Autodesk Fusion 360 part; units mm, degrees
sketch "main" plane through (0, 0, 0) normal (0, 1, 0) x (1, 0, 0) in component "crank-holder"
  line L0 (30, -20) -> (-30, -20)
  line L1 (-30, -20) -> (-30, 20)
  line L2 (-30, 20) -> (30, 20)
  line L3 (30, 20) -> (30, -20)
  line L4 (30, -20) -> (-30, 20) construction
  line L5 (-30, -20) -> (30, 20) construction
  circle A0 centre (0, 0) radius 4.425
  line L6 (-30, 20) -> (-50, 20) construction
  line L7 (-50, 20) -> (50, 20)
  line L8 (50, 20) -> (50, 5)
  line L9 (50, 5) -> (-50, 5)
  line L10 (-50, 5) -> (-50, 20)
  dimension "d1" = 60
  dimension "d2" = 40
  dimension "d3" = 8.85
  dimension "d4" = 20
  dimension "d5" = 100
  dimension "d6" = 15
extrude "Extrude1" add sketch "main" against normal blind 30 contours L0 L1 L3 L9 | L1 L2 L3 L7 L9 | L3 L7 L8 L9 | L1 L7 L9 L10 | A0 in component "crank-holder"
extrude "Extrude2" add sketch "main" along normal blind 8.5 contours A0 in component "crank-holder"
sketch "screws" plane through (0, 0, -5) normal (0, 0, 1) x (-1, 0, 0) in component "crank-holder"
  line L0 (30, 0) -> (50, 0)
  line L1 (50, 0) -> (50, 30)
  line L2 (50, 30) -> (30, 30)
  line L3 (30, 30) -> (30, 0)
  line L4 (50, 0) -> (30, 30) construction
  line L5 (50, 30) -> (30, 0) construction
  line L6 (-50, 0) -> (-30, 30) construction
  line L7 (-50, 30) -> (-30, 0) construction
  circle A0 centre (40, 15) radius 2.75
  circle A1 centre (-40, 15) radius 2.75
  point P0 (-50, 0)
  point P1 (-30, 30)
  point P2 (-50, 30)
  point P3 (-30, 0)
  dimension "d11" = 5.5
  dimension "d12" = 5.5
extrude "Extrude3" cut sketch "screws" against normal blind 15 contours A0 | A1 in component "crank-holder"
component "crank-holder" placed x (1, 0, 0) y (0, 1, 0) z (0, 0, 1) at (0, 0, 0)
equation "d5 = 20 mm + 60 mm + 20 mm"
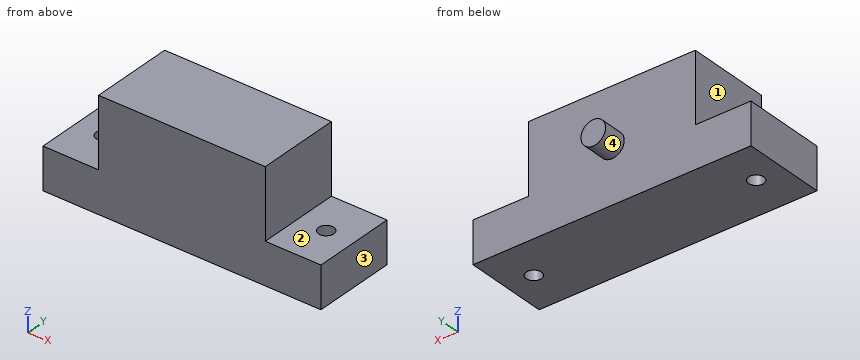
The listing builds one solid part. Answer for the finished solid, in the listing's coordinates (mm). Face numbers are marked on the shaded views. A direction names the side the tool comes from. Coordinates: 2 decimals unless noted, no trailing zeros. Loops run counter-clockwise (first coordinate to the right, second up) from the corner with the lowest first, then second, coordinate; pieces in that order, holes last. Notation, with made-up numbers: M 61,-39 L 85,-39 A14 ccw 85,-20 Z; hole C -35.75,62.5 d5. An arc over 180 degrees is marked long. Answer as a JSON object with one key per item and string values. Group by question number.
Item 1: Section C-C (z = 0) is taken. Write down the section's boundary in (x, y) (3 decimals).
Item 2: Consider L1, parallel to X at y = -15, z = -9.5; L2, parallel to Y at x = 40, z = -13.5; L3, parallel to Z at x = 37, y = -25.5. Determine where each line is inside the solid, lowest interval first.
Item 3: Which of the six approach directions +Z, -Z, +X, -X, +Y, -Y give full straight-line access (tool end or side, diameter ignored) to the marked faces 1, 2, 3 and 4?
Item 4: Section D-D (y = -7.5) is taken. Write down the section's boundary in (x, z), and give its area (3 significant figures).
Item 5: Section A-A (x = -40) is taken. Write down the section's boundary in (y, z).
Item 6: Section B-B (y = -15) is taken. Write down the section's boundary in (x, z), and give its area (4 significant figures).
Item 7: Each of these flat-tipped pins is pushed along its axis until it touches: P1, Ø6, axis at x = -35.5, y = -17.5, coming from the +Z side; P2, Ø7, axis at x = -40, y = -15, coming from the -Z side; P3, Ø10, axis at x = -3, z = -14, coming from the +Y side; P4, Ø1, axis at y = -10, z = 3.5, coming from the +X side. Where does it stop, or does it pass through?
Solved:
{
 "1": {"outline": "M -30,-30 L 30,-30 L 30,0 L 4.425,0 L 4.425,8.5 L -4.425,8.5 L -4.425,0 L -30,0 Z"},
 "2": {"L1": "x = -50 to -42.75, -37.25 to 37.25, 42.75 to 50", "L2": "y = -30 to -17.75, -12.25 to 0", "L3": "z = -20 to -5"},
 "3": {"face 1": "+Z, -X, +Y, -Y", "face 2": "+Z, +X, +Y, -Y", "face 3": "+Z, -Z, +X, +Y, -Y", "face 4": "+Y"},
 "4": {"outline": "M -50,-20 L 50,-20 L 50,-5 L 30,-5 L 30,20 L -30,20 L -30,-5 L -50,-5 Z", "area": "3,000 mm2"},
 "5": {"outline": "M -30,-20 L -17.75,-20 L -17.75,-5 L -30,-5 Z; M -12.25,-20 L 0,-20 L 0,-5 L -12.25,-5 Z"},
 "6": {"outline": "M -50,-20 L -42.75,-20 L -42.75,-5 L -50,-5 Z; M -37.25,-20 L 37.25,-20 L 37.25,-5 L 30,-5 L 30,20 L -30,20 L -30,-5 L -37.25,-5 Z; M 42.75,-20 L 50,-20 L 50,-5 L 42.75,-5 Z", "area": "2,835 mm2"},
 "7": {"P1": "stops at z = -5", "P2": "stops at z = -20", "P3": "stops at y = 0", "P4": "stops at x = 30"}
}
